The model under review builds one solid part; all positions refer to its coordinate system, in mm. A direction names the side the tool comes from. Round coordinates to 2 decimals unless told otherwise and drop trailing zeros. Loops run counter-clockwise (first coordinate to the right, second up) from the corner with the lowest first, then second, coordinate; pieces in that order, holes last. Notation, with made-up numbers: (42, 65.5) -> (91, 65.5) arc R20 cw to (91, 75.5) -> close; hole circle Ø11 at (-12.5, -26.75). An arc over 180 degrees is marked (long way). Use a Markdown table: item, result. Add a question column.
1) Wall thickness on probe 1 along X at (y, z) = (3.75, -54); probe 2 along X at (y, z) = (1.3, -42); probe 3 along Z at (x, y) = (62, 3.5): over which ranges is each line inside the solid? List them lowest first.
2) Mouldability with a two-part tool opening along Z and no side actions: class faces 1 (the flat face through (123, 2, -55)), 2 (the flat face through (138, 2, -75)), 3 (the flat face through (75, 3, -15)) as released by +Z, released by -Z, zero draft, split by the parting line, or undercut.
3) Consider section A-A on x = 82. Give the boundary of the cut face in (y, z).
4) Consider section C-C on z = -62.5. Give the boundary of the cut face in (x, y), plus the area to 3 significant figures.
5) For faces 4 (the flat face through (83, 2, 0)), 5 (the flat face through (13, 2, -20)), 6 (the flat face through (137, 2, -55)), 7 (the cylindrical face through (95.15, 2.46, -56.99)), list the 3-axis set-ups (+Z, -Z, +X, -X, +Y, -Y) from which the entire face can be reached by the end or side of a thin tool; tool diameter is ignored.
6) Consider section B-B on y = 1.95. Give the boundary of the cut face in (x, z), plus the area to 3 significant figures.
7) Consider section D-D on z = -22. Give the boundary of the cut face in (x, y).
from build123d import *

# Parameters (mm, degrees)
SKETCH2_W               = 150
SKETCH2_H               = 75
BOSS_EXTRUDE1_DEPTH     = 5
CUT_EXTRUDE1_DEPTH      = 168.779617356
CUT_EXTRUDE1_DEPTH_BACK = 168.779617356
SKETCH4_W               = 46
SKETCH4_H               = 45
CUT_EXTRUDE2_DEPTH      = 168.779617356
FILLET1_R               = 10
FILLET2_R               = 10


with BuildPart() as part:
    # Sketch2 → Boss-Extrude1 (new body)
    with BuildSketch(Plane(origin=(0, 0, 0), x_dir=(1, 0, 0), z_dir=(0, 1, 0))):
        with Locations((75, 37.5)):
            Rectangle(SKETCH2_W, SKETCH2_H)
    extrude(amount=BOSS_EXTRUDE1_DEPTH)

    # Sketch3 → Cut-Extrude1 (cut, two sides: drawn at the far end of the back side and taken through both)
    with BuildSketch(Plane(origin=(0, 5, 0), x_dir=(1, 0, 0), z_dir=(0, 1, 0)).offset(-CUT_EXTRUDE1_DEPTH_BACK)):
        with BuildLine():
            Line((13, 0), (13, 40))
            ThreePointArc((13, 40), (20, 47), (27, 40))
            Line((27, 40), (27, 0))
            Line((27, 0), (13, 0))
        make_face()
        with BuildLine():
            Line((137, 75), (137, 35))
            ThreePointArc((137, 35), (130, 28), (123, 35))
            Line((123, 35), (123, 75))
            Line((123, 75), (137, 75))
        make_face()
    extrude(amount=CUT_EXTRUDE1_DEPTH + CUT_EXTRUDE1_DEPTH_BACK, mode=Mode.SUBTRACT)

    # Sketch4 → Cut-Extrude2 (cut, through all)
    with BuildSketch(Plane(origin=(0, 5, 0), x_dir=(1, 0, 0), z_dir=(0, 1, 0))):
        with Locations((75, 37.5)):
            Rectangle(SKETCH4_W, SKETCH4_H)
    extrude(amount=-CUT_EXTRUDE2_DEPTH, mode=Mode.SUBTRACT)

    # Fillet1
    fillet1_edges = [part.edges().sort_by_distance(p)[0] for p in [
        (0, 2.5, 0),
        (0, 2.5, -75),
        (150, 2.5, -75),
        (150, 2.5, 0),
    ]]
    fillet(fillet1_edges, radius=FILLET1_R)

    # Fillet2
    fillet2_edges = [part.edges().sort_by_distance(p)[0] for p in [
        (52, 2.5, -15),
        (52, 2.5, -60),
        (98, 2.5, -60),
        (98, 2.5, -15),
    ]]
    fillet(fillet2_edges, radius=FILLET2_R)


solid = part.part
Result set:
| question | item | result |
|---|---|---|
| 1 | probe 1 | 0 to 52.83, 97.17 to 123, 137 to 150 |
| 1 | probe 2 | 0 to 13.29, 26.71 to 52, 98 to 123, 137 to 150 |
| 1 | probe 3 | -75 to -60, -15 to 0 |
| 2 | face 1 | zero draft |
| 2 | face 2 | released by -Z |
| 2 | face 3 | undercut |
| 3 | outline | (0, -75) -> (5, -75) -> (5, -60) -> (0, -60) -> close; (0, -15) -> (5, -15) -> (5, 0) -> (0, 0) -> close |
| 4 | outline | (0, 0) -> (123, 0) -> (123, 5) -> (0, 5) -> close; (137, 0) -> (150, 0) -> (150, 5) -> (137, 5) -> close |
| 4 | area | 680 mm2 |
| 5 | face 4 | +Z, +X, -X, +Y, -Y |
| 5 | face 5 | +Z, +Y, -Y |
| 5 | face 6 | -Z, +Y, -Y |
| 5 | face 7 | +Y, -Y |
| 6 | outline | (0, -65) arc R10 ccw to (10, -75) -> (123, -75) -> (123, -35) arc R7 cw to (137, -35) -> (137, -75) -> (140, -75) arc R10 ccw to (150, -65) -> (150, -10) arc R10 ccw to (140, 0) -> (27, 0) -> (27, -40) arc R7 cw to (13, -40) -> (13, 0) -> (10, 0) arc R10 ccw to (0, -10) -> close; hole (52, -50) arc R10 ccw to (62, -60) -> (88, -60) arc R10 ccw to (98, -50) -> (98, -25) arc R10 ccw to (88, -15) -> (62, -15) arc R10 ccw to (52, -25) -> close |
| 6 | area | 7,910 mm2 |
| 7 | outline | (0, 0) -> (13, 0) -> (13, 5) -> (0, 5) -> close; (27, 0) -> (52.46, 0) -> (52.46, 5) -> (27, 5) -> close; (97.54, 0) -> (150, 0) -> (150, 5) -> (97.54, 5) -> close |
